Autodesk Inventor part; units mm, degrees
ref_plane "YZ Plane" through (0, 0, 0) normal (1, 0, 0) x (0, 1, 0)
ref_plane "XZ Plane" through (0, 0, 0) normal (0, 1, 0) x (-1, 0, 0)
ref_plane "XY Plane" through (0, 0, 0) normal (0, 0, 1) x (1, 0, 0)
sketch "Sketch1" plane through (0, 0, 0) normal (0, 0, 1) x (1, 0, 0)
  line L0 (0, 0) -> (292.1, 0)
  line L1 (292.1, 0) -> (292.1, 3.175)
  line L2 (292.1, 3.175) -> (0, 3.175)
  line L3 (0, 3.175) -> (0, 0)
  dimension "d0" = 292.1
  dimension "d1" = 3.175
extrude "Extrusion1" add sketch "Sketch1" along normal blind 139.7
sketch "Sketch2" plane through (0, 3.175, 0) normal (0, 1, 0) x (1, 0, 0)
  point P0 (0, 0)
  point P1 (96.8502, -31.75)
  point P2 (96.8502, -95.75)
  point P3 (182.5498, -31.75)
  point P4 (182.5498, -95.75)
  dimension "d4" = 64
  dimension "d5" = 31.75
  dimension "d6" = 64
  dimension "d7" = 31.75
  dimension "d15" = 85.6996
  dimension "d16" = 85.6996
  dimension "d17" = 96.8502
  dimension "d18" = 96.8502
hole "Hole1" at (96.8502, 3.175, 31.75) at (96.8502, 3.175, 95.75) at (182.5498, 3.175, 31.75) at (182.5498, 3.175, 95.75) direction (0, -1, 0) diameter 4.1656 end through all
sketch "Sketch3" plane through (0, 3.175, 0) normal (0, 1, 0) x (1, 0, 0)
  line L0 (111.125, -38.1) -> (168.275, -38.1)
  line L1 (168.275, -38.1) -> (168.275, -101.6)
  line L2 (168.275, -101.6) -> (111.125, -101.6)
  line L3 (111.125, -101.6) -> (111.125, -38.1)
  line L4 (292.1, -139.7) -> (0, -139.7)
  point P0 (0, 0)
  dimension "d19" = 57.15
  dimension "d20" = 63.5
  dimension "d24" = 111.125
  dimension "d26" = 38.1
extrude "Extrusion2" cut sketch "Sketch3" against normal blind 25.4
properties part number "Winch baseplate"
Input: part model. Units: mm. Frame: model coordinates. Give positions to 0.01 mm unless a question says otherwise; leave off trailing zeros. Order: outer loops, then holes, each group sorted by start corner. A loop starts at its lowest first (then second) coordinate and runs counter-clockwise, first axis right, second up. Notation, with made-up numbers: M 72,-28.5 L 120,-28.5 A19 cw 120,-23.5 Z; hole C 25,-5 d4. An arc over 180 degrees is marked long. Return JSON: item names as keys, results as strings.
1) Section query B-B on y = 1.55. Output: boundary loops of the cut face in (x, z) (3 decimals).
Taken from the geometry:
{"outline": "M 0,0 L 292.1,0 L 292.1,139.7 L 0,139.7 Z; hole C 96.85,31.75 d4.166; hole C 96.85,95.75 d4.166; hole M 111.125,38.1 L 168.275,38.1 L 168.275,101.6 L 111.125,101.6 Z; hole C 182.55,31.75 d4.166; hole C 182.55,95.75 d4.166"}
2) Line query: L1, parallel to X at y = 1.85, z = 95.75 (3 decimals); L2, parallel to X at y = 2.45, z = 31.75; L3, parallel to X at y = 0.2, z = 70 (3 decimals). Output: solid intervals per line, ascending. Write a range as [from, to].
Taken from the geometry:
{"L1": "x = [0, 94.767], [98.933, 111.125], [168.275, 180.467], [184.633, 292.1]", "L2": "x = [0, 94.77], [98.93, 180.47], [184.63, 292.1]", "L3": "x = [0, 111.125], [168.275, 292.1]"}
3) Section query A-A on z = 83. Output: boundary loops of the cut face in (x, y) (3 decimals).
Taken from the geometry:
{"outline": "M 0,0 L 111.125,0 L 111.125,3.175 L 0,3.175 Z; M 168.275,0 L 292.1,0 L 292.1,3.175 L 168.275,3.175 Z"}
4) Mould query, pull axis Y, two halves, no side actions, for faces 1 (the face through (144, 0, 37.8)), 2 (the face through (148.1, 3.175, 37.8)). Classes: released by +Y, released by -Y, zero draft, split by the parting line, or undercut.
Taken from the geometry:
{"face 1": "released by -Y", "face 2": "released by +Y"}
